Check sheet for the drawn part. Datum: minimum x, y, z corner. Units: mm. A direction names the side the tool comes from. Coordinates: 2 decimals unless noted, no trailing zeros. Write each loop counter-clockwise with the first axis right and the second up, starting at its lowest first coordinate (ties: lowest second). Pieces come first, ordered by that corner, then holes. Notation, with made-up numbers: (59.5, 14) - (64.5, 14) arc R16 cw to (64.5, 37) - close; hole circle Ø11 at (-4, -20.5). An arc over 180 degrees is marked (long way). Use one line per item in the form item = value. Start each with the question number.
1. Cross-section at B-B on z = 58. Record the boundary of the cut face in (x, y), then the cut area to 3 significant figures.
2. Draft check along X on the marked faces 3 and 4. Enter one of: +X half, -X half, draft (parallel to the pull), parting line (faces both ways), or undercut.
3. Tool access check on the marked faces 1 and 2. Record the directions out of +Z, -Z, +X, -X, +Y, -Y that give a thin tool (end or side, any length) a straight path to the whole face; none if there is none.
4. Go/stop test with flat-tipped pins: pin 1 Ø2 at (y, z) = (3, 51.5) entering from -X; pin 2 Ø2.5 at (y, z) = (7, 63.5) entering from -X; pin 3 Ø1.5 at (x, y) = (102.5, 7.5) entering from -Z. Record where each tip stops, or that it passes through.
5. Cross-section at D-D on x = 23.5. Record the boundary of the cut face in (y, z) (1 decimal).
6. Cross-section at C-C on y = 2.25. Record the boundary of the cut face in (x, z).
7. Scan lines: line 1 along X through (y, z) = (8.5, 56); line 2 along Y through (x, z) = (87.5, 55.5); line 3 along X through (y, z) = (2.75, 108.5). Record each from-to range of solid material in increasing order.
8. Cross-section at A-A on x = 99. Record the boundary of the cut face in (y, z).
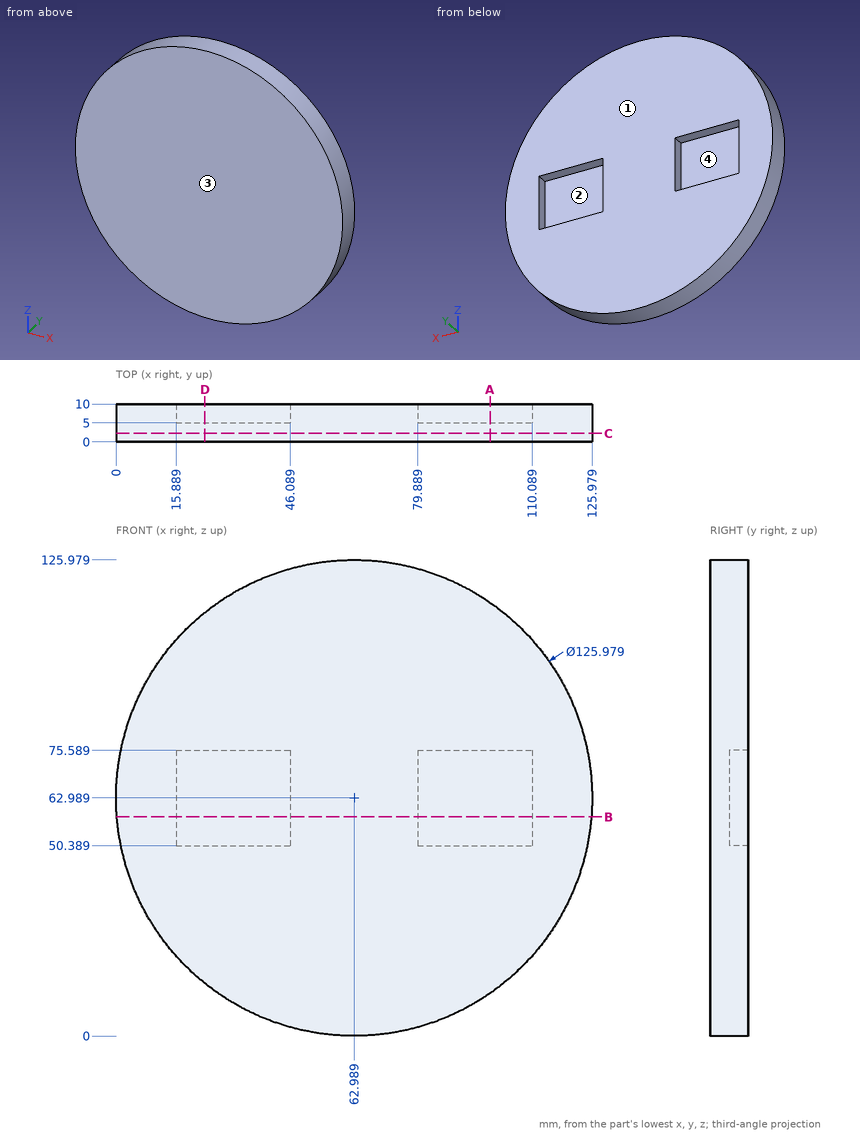
Final values:
q1.outline = (0.2, 0) - (125.78, 0) - (125.78, 10) - (110.09, 10) - (110.09, 5) - (79.89, 5) - (79.89, 10) - (46.09, 10) - (46.09, 5) - (15.89, 5) - (15.89, 10) - (0.2, 10) - close
q1.area = 954 mm²
q2.face_3 = draft
q2.face_4 = undercut
q3.face_1 = +Z, -Z, +X, -X, +Y
q3.face_2 = +Y
q4.pin_1 = 0.88
q4.pin_2 = 0
q4.pin_3 = 13.34
q5.outline = (0, 13.9) - (10, 13.9) - (10, 50.4) - (5, 50.4) - (5, 75.6) - (10, 75.6) - (10, 112.1) - (0, 112.1) - close
q6.outline = circle Ø125.98 at (62.99, 62.99)
q7.line_1 = 0.39 to 15.89, 46.09 to 79.89, 110.09 to 125.59
q7.line_2 = 0 to 5
q7.line_3 = 19.44 to 106.54
q8.outline = (0, 11.31) - (10, 11.31) - (10, 50.39) - (5, 50.39) - (5, 75.59) - (10, 75.59) - (10, 114.67) - (0, 114.67) - close
